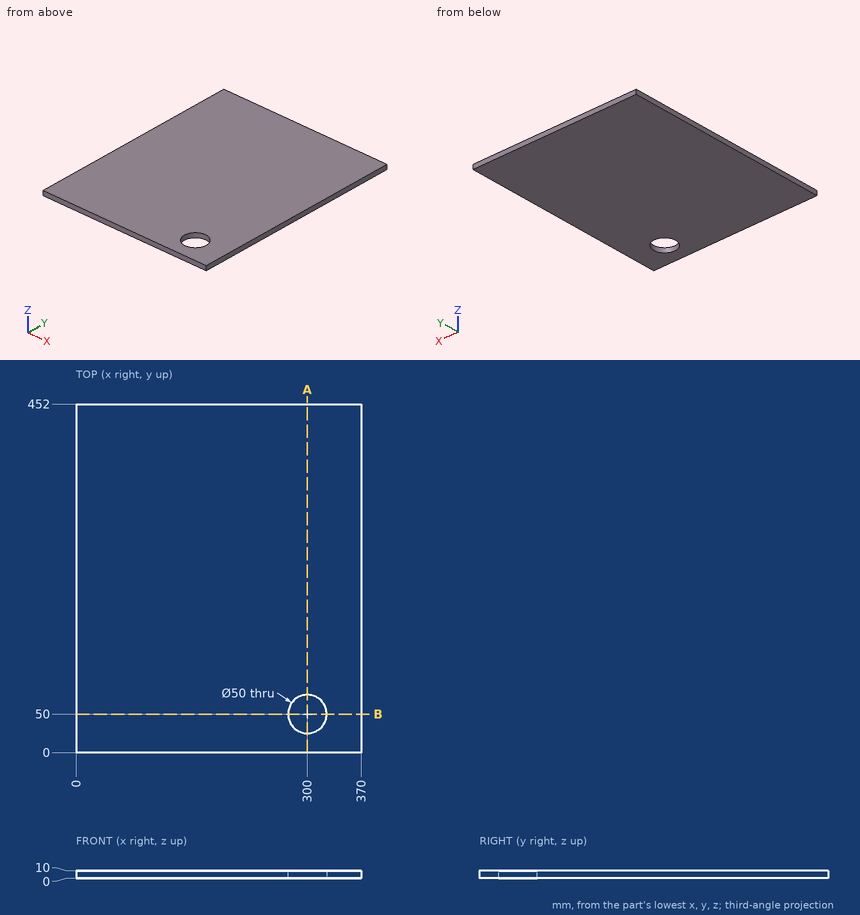
Source: three-view drawing plus pictorial views. Frame: mm from the lowest corner of the part. Give positions to 0.01 mm unless a question says otherwise; leave off trailing zeros. Write each loop counter-clockwise with the first axis right and the second up, starting at its lowest first coordinate (ties: lowest second). Pieces come first, ordered by that corner, then holes. Notation, with made-up numbers: (89, 48.5) - (100, 48.5) arc R28 ccw to (100, 86.5) - close; hole circle Ø3 at (28.25, 34.25). An arc over 180 degrees is marked (long way). Write item = value, one per line. Start each with the question number.
Q1. Material intervals for probe 1 along X at (y, z) = (52, 6.25); probe 2 along Y at (x, z) = (300, 5.5); probe 3 along X at (y, z) = (69.5, 8.25), sorted ascending.
Q2. Cut plane A-A, the plane x = 300. Return loops of the section in (y, z).
Q3. Cut plane B-B, the plane y = 50. Return loops of the section in (x, z).
Computed values:
q1.probe_1 = 0 to 275.08, 324.92 to 370
q1.probe_2 = 0 to 25, 75 to 452
q1.probe_3 = 0 to 284.36, 315.64 to 370
q2.outline = (0, 0) - (25, 0) - (25, 10) - (0, 10) - close; (75, 0) - (452, 0) - (452, 10) - (75, 10) - close
q3.outline = (0, 0) - (275, 0) - (275, 10) - (0, 10) - close; (325, 0) - (370, 0) - (370, 10) - (325, 10) - close
